```python
from build123d import *

# Parameters (mm, degrees)
BOSS_EXTRUDE1_DEPTH      = 1.5
SKETCH2_R                = 6
SKETCH2_W                = 16
SKETCH2_H                = 4
CUT_EXTRUDE1_DEPTH       = 2
SKETCH3_W                = 57
SKETCH3_H                = 37
SKETCH3_W_2              = 54
SKETCH3_H_2              = 34
BOSS_EXTRUDE2_DEPTH      = 15
BOSS_EXTRUDE2_DEPTH_BACK = 1.5
FILLET1_R                = 2


with BuildPart() as part:
    # Sketch1 → Boss-Extrude1 (new body)
    with BuildSketch(Plane.XY):
        Polygon((-27, -17), (-7.5, -17), (7.5, -17), (27, -17), (27, 17), (-27, 17), align=None)
    extrude(amount=BOSS_EXTRUDE1_DEPTH)

    # Sketch2 → Cut-Extrude1 (cut)
    with BuildSketch(Plane.XY.offset(1.5)):
        with Locations((-17, -5)):
            Circle(SKETCH2_R)
        with Locations((15, 10.5)):
            Rectangle(SKETCH2_W, SKETCH2_H)
    extrude(amount=-CUT_EXTRUDE1_DEPTH, mode=Mode.SUBTRACT)

    # Sketch3 → Boss-Extrude2 (add, two sides)
    with BuildSketch(Plane(origin=(0, 0, 0), x_dir=(-1, 0, 0), z_dir=(0, 0, -1))) as boss_extrude2_sk:
        Rectangle(SKETCH3_W, SKETCH3_H)
        Rectangle(SKETCH3_W_2, SKETCH3_H_2, mode=Mode.SUBTRACT)
    extrude(amount=BOSS_EXTRUDE2_DEPTH)
    extrude(boss_extrude2_sk.sketch, amount=-BOSS_EXTRUDE2_DEPTH_BACK)

    # Fillet1
    fillet1_edges = [part.edges().sort_by_distance(p)[0] for p in [
        (28.5, -18.5, -6.75),
        (28.5, 0, 1.5),
        (28.5, 18.5, -6.75),
        (0, 18.5, 1.5),
        (-28.5, 18.5, -6.75),
        (-28.5, 0, 1.5),
        (-28.5, -18.5, -6.75),
        (0, -18.5, 1.5),
    ]]
    fillet(fillet1_edges, radius=FILLET1_R)


solid = part.part
```
CAD build for the part. Positions are in the model's coordinates, mm. A direction names the side the tool comes from. Round coordinates to 2 decimals unless told otherwise and drop trailing zeros. Loops run counter-clockwise (first coordinate to the right, second up) from the corner with the lowest first, then second, coordinate; pieces in that order, holes last. Notation, with made-up numbers: M -23,5.5 L 31,5.5 A8 ccw 31,17.5 Z; hole C -20,81 d2. An arc over 180 degrees is marked long. Return JSON: item names as keys, results as strings. Group by question number.
(1) Saw through at A-A, the plane y = -5. List the corners of the cut face in (x, z), and give its area (3 significant figures).
(2) Mould opens along Y. For faces 1 (the flat face through (23, 10, 1)), 2 (the cylindrical face through (27.93, 17.9, -7.65)), 3 (the cylindrical face through (27.93, 0.23, 0.9)) say: +Y half, -Y half, draft (parallel to the pull), parting line (faces both ways), or undercut.
(3) Wall check: probe 1 along X at (y, z) = (-10.5, -1.5); probe 2 along Y at (x, z) = (24.5, -6.5); probe 3 along Z at (x, y) = (8.5, -3.5). Give the ranges that are in metal, low to high. Write a range as [from, to].
(4) Saw through at C-C, the plane z = -4.25. List the corners of the cut face in (x, y), and give its area (3 significant figures).
(5) Saw through at B-B, the plane x = -17. List the corners of the cut face in (y, z).
(6) Tool access for faces 4 (the cylindrical face through (27.93, -17.9, -7.85)), 5 (the flat face through (-27, 0, -7)), 6 (the flat face through (15, 12.5, 1)): list every direction of +Z, -Z, +X, -X, +Y, -Y with a clear straight run to the whole face (end or side of a thin tool).
(7) Drop flat-ended pins along their axis: P1, Ø1.2, axis at y = 10, z = 1, coming from the +X side; P2, Ø1.6, axis at y = 10.5, z = 1, coming from the -X side; P3, Ø10, axis at x = -7.5, y = -3.5, coming from the -Z side. Give the stop position or say it passes through.
(8) Saw through at D-D, the plane x = -4. List the corners of the cut face in (y, z), and give its area (3 significant figures).
Answer list:
{
 "1": {"outline": "M -28.5,-15 L -27,-15 L -27,0 L -23,0 L -23,1.5 L -26.5,1.5 A2 ccw -28.5,-0.5 Z; M -11,0 L 27,0 L 27,-15 L 28.5,-15 L 28.5,-0.5 A2 ccw 26.5,1.5 L -11,1.5 Z", "area": "111 mm2"},
 "2": {"face 1": "undercut", "face 2": "+Y half", "face 3": "draft"},
 "3": {"probe 1": "[-28.5, -27], [27, 28.5]", "probe 2": "[-18.5, -17], [17, 18.5]", "probe 3": "[0, 1.5]"},
 "4": {"outline": "M -28.5,-16.5 A2 ccw -26.5,-18.5 L 26.5,-18.5 A2 ccw 28.5,-16.5 L 28.5,16.5 A2 ccw 26.5,18.5 L -26.5,18.5 A2 ccw -28.5,16.5 Z; hole M -27,-17 L 27,-17 L 27,17 L -27,17 Z", "area": "270 mm2"},
 "5": {"outline": "M -18.5,-15 L -17,-15 L -17,0 L -11,0 L -11,1.5 L -16.5,1.5 A2 ccw -18.5,-0.5 Z; M 1,0 L 17,0 L 17,-15 L 18.5,-15 L 18.5,-0.5 A2 ccw 16.5,1.5 L 1,1.5 Z"},
 "6": {"face 4": "+Z, -Z, +X, -Y", "face 5": "-Z", "face 6": "+Z, -Z"},
 "7": {"P1": "x = 28.29", "P2": "x = -28.37", "P3": "z = 0"},
 "8": {"outline": "M -18.5,-15 L -17,-15 L -17,0 L 17,0 L 17,-15 L 18.5,-15 L 18.5,-0.5 A2 ccw 16.5,1.5 L -16.5,1.5 A2 ccw -18.5,-0.5 Z", "area": "98.8 mm2"}
}
